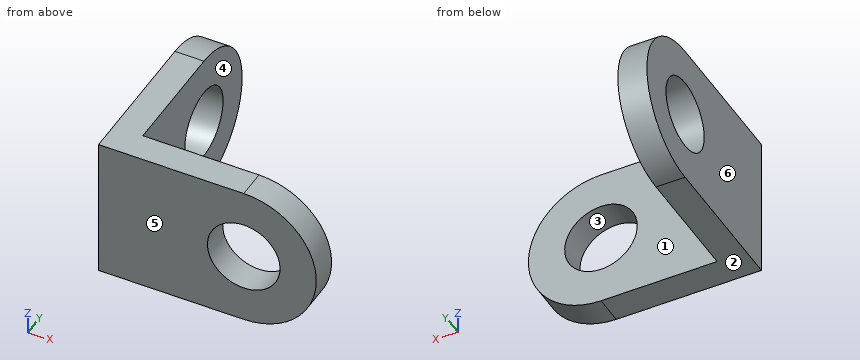
from build123d import *

# Parameters (mm, degrees)
ESBO_O1_R                = 5
ESBO_O1_R_2              = 2.5
RESSALTO_EXTRUS_O1_DEPTH = 2
ESBO_O2_R                = 2.5
RESSALTO_EXTRUS_O2_DEPTH = 2


with BuildPart() as part:
    # Esboço1 → Ressalto-extrusão1 (new body)
    # profile 1 of 2: a face of its own
    with BuildSketch(Plane(origin=(0, 0, 0), x_dir=(1, 0, 0), z_dir=(0, 1, 0))):
        with BuildLine():
            ThreePointArc((0, -5), (-5, 0), (0, 5))
            Line((0, 5), (-10, 5))
            Line((-10, 5), (-10, -5))
            Line((-10, -5), (0, -5))
        make_face()
    # profile 2 of 2: a face of its own
    with BuildSketch(Plane(origin=(0, 0, 0), x_dir=(1, 0, 0), z_dir=(0, 1, 0))):
        Circle(ESBO_O1_R)
        with Locations(Location((0, 0, 0), (0, 0, 270))):
            Circle(ESBO_O1_R_2, mode=Mode.SUBTRACT)
    extrude(amount=RESSALTO_EXTRUS_O1_DEPTH)

    # Esboço2 → Ressalto-extrusão2 (add)
    with BuildSketch(Plane.ZY.offset(10)):
        with BuildLine():
            ThreePointArc((5, 10), (0, 15), (-5, 10))
            Line((-5, 10), (-5, 2))
            Line((-5, 2), (5, 2))
            Line((5, 2), (5, 10))
        make_face()
        with Locations((0, 10)):
            Circle(ESBO_O2_R, mode=Mode.SUBTRACT)
    extrude(amount=-RESSALTO_EXTRUS_O2_DEPTH)


solid = part.part
The listing builds one solid part. Answer for the finished solid, in the listing's coordinates (mm). Face numbers are marked on the shaded views. A direction names the side the tool comes from. Round coordinates to 2 decimals unless told otherwise and drop trailing zeros. Write each loop counter-clockwise with the first axis right and the second up, starting at its lowest first coordinate (ties: lowest second). Pieces come first, ordered by that corner, then holes. Notation, with made-up numbers: M -39.75,20 L -3.75,20 A37 ccw -3.75,57 Z; hole C -21,-17 d5. An arc over 180 degrees is marked long. Write each question's results on one line, items separated by ' | '. Start each with the question number.
(1) The part is cut by section A-A, the plane z = 0. Write down the section's boundary in (x, y).
(2) For the marked faces 1 and 2, determine the directions among +Z, -Z, +X, -X, +Y, -Y from which every point of the face is accessible in a straight line to the end or side of a thin tool.
(3) The part is cut by section B-B, the plane x = -2. Write down the section's boundary in (y, z).
(4) The part is cut by section C-C, the plane x = -8.25. Write down the section's boundary in (y, z), and give its area (3 significant figures).
(5) Each of these flat-tipped pins is pushed along its axis until it touches: P1, Ø1, axis at x = -2.5, z = -2.5, coming from the -Y side; P2, Ø1, axis at y = 5, z = -2.5, coming from the +X side; P3, Ø5, axis at x = 1, z = 3, coming from the +Y side. Where does it stop, or does it pass through?
(6) The part is cut by section D-D, the plane y = 4.75. Write down the section's boundary in (x, z), and give its area (3 significant figures).
(7) Find the intervals of material crossed by line 1 (Y direction, x = -9.35, z = 0); line 2 (Y direction, x = 1.75, z = 4.25); line 3 (X direction, y = 3, z = -2.5), in increasing order.
(8) Determine the mould class of the marked faces 3, 4, 5 and 6 for opening direction X: +X half, -X half, draft (parallel to the pull), parting line (faces both ways), or undercut.
Worked answers:
1) outline: M -10,0 L -2.5,0 L -2.5,2 L -8,2 L -8,7.5 L -10,7.5 Z; M -10,12.5 L -8,12.5 L -8,15 L -10,15 Z; M 2.5,0 L 5,0 L 5,2 L 2.5,2 Z
2) face 1: +Z, -Z, +X, +Y | face 2: -Z, +X, -X, +Y, -Y
3) outline: M 0,-5 L 2,-5 L 2,-1.5 L 0,-1.5 Z; M 0,1.5 L 2,1.5 L 2,5 L 0,5 Z
4) outline: M 0,-5 L 10,-5 A5 ccw 10,5 L 0,5 Z; hole C 10,0 d5 | area: 120 mm²
5) P1: stops at y = 0 | P2: stops at x = -8 | P3: stops at y = 2
6) outline: M -10,-5 L -8,-5 L -8,5 L -10,5 Z | area: 20.0 mm²
7) line 1: y = 0 to 7.5, 12.5 to 15 | line 2: y = 0 to 2 | line 3: x = -10 to -8
8) face 3: undercut | face 4: +X half | face 5: draft | face 6: -X half
